Model file for the job. Use its own axes, mm. Face numbers are marked on the shaded views. A direction names the side the tool comes from. Coordinates: 2 decimals unless noted, no trailing zeros. Write each loop counter-clockwise with the first axis right and the second up, starting at its lowest first coordinate (ties: lowest second). Pieces come first, ordered by that corner, then holes. Notation, with made-up numbers: (38.5, 89.5) -> (48.5, 89.5) arc R27 cw to (48.5, 122.5) -> close; hole circle Ø4 at (30, 79). An arc over 180 degrees is marked (long way). Answer as a JSON object with one key per item and string values. Group by question number.
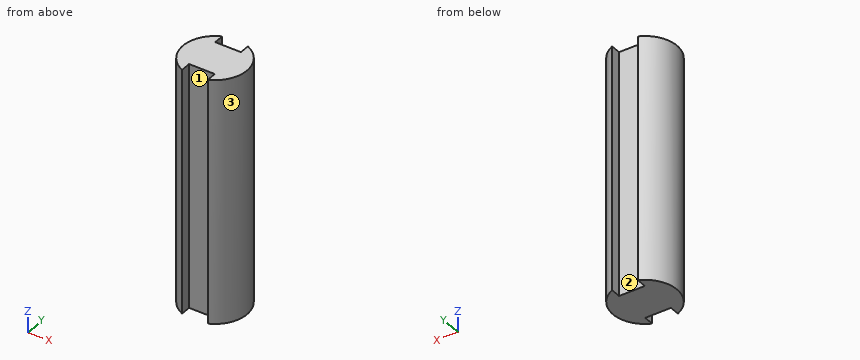
Autodesk Inventor part; units mm, degrees
ref_plane "YZ Plane" through (0, 0, 0) normal (1, 0, 0) x (0, 1, 0)
ref_plane "XZ Plane" through (0, 0, 0) normal (0, 1, 0) x (-1, 0, 0)
ref_plane "XY Plane" through (0, 0, 0) normal (0, 0, 1) x (1, 0, 0)
sketch "Sketch1" plane through (0, 0, 0) normal (0, 0, 1) x (1, 0, 0)
  circle A0 centre (0, 0) radius 3.925
  line L0 (-1.575, 5.5) -> (1.575, 5.5)
  line L1 (1.575, 5.5) -> (1.575, 2.35)
  line L2 (1.575, 2.35) -> (-1.575, 2.35)
  line L3 (-1.575, 2.35) -> (-1.575, 5.5)
  line L4 (-1.575, 5.5) -> (1.575, 2.35) construction
  line L5 (1.575, 5.5) -> (-1.575, 2.35) construction
  line L6 (-1.575, -5.5) -> (1.575, -5.5)
  line L7 (1.575, -5.5) -> (1.575, -2.35)
  line L8 (1.575, -2.35) -> (-1.575, -2.35)
  line L9 (-1.575, -2.35) -> (-1.575, -5.5)
  line L10 (-1.575, -5.5) -> (1.575, -2.35) construction
  line L11 (1.575, -5.5) -> (-1.575, -2.35) construction
  point P0 (0, 3.925)
  point P1 (0, -3.925)
  point P2 (-1.575, 3.5951)
  point P3 (-1.575, -3.5951)
  point P4 (1.575, -3.5951)
  point P5 (1.575, 3.5951)
  dimension "d0" = 7.85
  dimension "d1" = 3.15
  dimension "d2" = 3.15
  dimension "d3" = 3.15
  dimension "d4" = 3.15
extrude "Extrusion1" add sketch "Sketch1" along normal blind 30 contours A0 L7 L8 L9 L3 L2 L1
properties part number "long_axel"
(1) Cut at D-D on y = 1.25. List the corners of the cut face in (x, z).
(2) Pin check, flat tips, straight feed: pin 1 (1 mm diameter, centred on y = 3, z = 19, fed in from +X); pin 2 (2 mm diameter, centred on x = 2, z = 25.5, fed in from +Y); pin 3 (1 mm diameter, centred on y = 3, z = 17, fed in from -X). Stop position of each tip, or through.
(3) Cut at C-C on x = -1. List the corners of the cut face in (y, z).
(4) Cut at B-B on z = 9. List the corners of the cut face in (x, y) (3 decimals), plus the area to 3 significant figures.
(5) Wall check: probe 1 along Y at (x, z) = (0, 28.5); probe 2 along X at (y, z) = (2.75, 27.75) (3 decimals); probe 3 along X at (y, z) = (2.5, 28.25) (3 decimals). Give the ranges that are in metal, low to high.
(6) 3-axis set-ups, long thin cutter, end or side, ignore diameter. For the marked faces 1, 2 and 3: which of +Z, -Z, +X, -X, +Y, -Y reach the whole face in a straight line?
(7) Cut at A-A on y = 3.25. List the corners of the cut face in (x, z) (3 decimals).
Results found:
{
 "1": {"outline": "(-3.72, 0) -> (3.72, 0) -> (3.72, 30) -> (-3.72, 30) -> close"},
 "2": {"pin 1": "stops at x = 3.03", "pin 2": "stops at y = 3.6", "pin 3": "stops at x = -3.03"},
 "3": {"outline": "(-2.35, 0) -> (2.35, 0) -> (2.35, 30) -> (-2.35, 30) -> close"},
 "4": {"outline": "(-1.575, -3.595) -> (-1.575, -2.35) -> (1.575, -2.35) -> (1.575, -3.595) arc R3.925 ccw to (1.575, 3.595) -> (1.575, 2.35) -> (-1.575, 2.35) -> (-1.575, 3.595) arc R3.925 ccw to start", "area": "39.2 mm²"},
 "5": {"probe 1": "y = -2.35 to 2.35", "probe 2": "x = -2.801 to -1.575, 1.575 to 2.801", "probe 3": "x = -3.026 to -1.575, 1.575 to 3.026"},
 "6": {"face 1": "+Z, -Z, -Y", "face 2": "+Z, -Z, +Y", "face 3": "+Z, -Z, +X"},
 "7": {"outline": "(-2.201, 0) -> (-1.575, 0) -> (-1.575, 30) -> (-2.201, 30) -> close; (1.575, 0) -> (2.201, 0) -> (2.201, 30) -> (1.575, 30) -> close"}
}
